Part model, mm, in its own coordinate system. A direction names the side the tool comes from. Coordinates: 2 decimals unless noted, no trailing zeros. Loops run counter-clockwise (first coordinate to the right, second up) from the corner with the lowest first, then second, coordinate; pieces in that order, holes last. Notation, with made-up numbers: M 9,47 L 62,47 A22 cw 62,59 Z; hole C 56.5,-28.75 d5. An arc over 180 degrees is marked long. Answer as a JSON object with one key per item and string values. Group by question number.
1. Saw through at B-B on z = 68.5. Write the cut outline in (x, y), then the cut area to 3 significant figures.
2. Saw through at C-C on z = 104. Write the cut outline in (x, y), then the cut area to 3 significant figures.
3. Drop flat-ended pins along their axis: pin 1 Ø5 at (x, z) = (-1, -143.5) entering from +Y; pin 2 Ø2 at (y, z) = (-1.5, 30.5) entering from +X; pin 3 Ø1.5 at (y, z) = (-4, -95.5) entering from -X. Give the stop position or say it passes through.
4. Saw through at A-A on x = 0. Write the cut outline in (y, z), then the cut area to 3 significant figures.
5. 3-axis set-ups, long thin cutter, end or side, ignore diameter. For faces 1 (the face through (11, 2, 74)), 2 (the face through (0, 8, -145)), 3 (the face through (11, 2, -74)), 4 (the face through (0, 0, 159)): which of +Z, -Z, +X, -X, +Y, -Y reach the whole face in a straight line?
6. Drill centre lines: L1, parallel to Z at x = 6, y = -13; L2, parallel to Y at x = 11.5, z = 42; L3, parallel to X at y = -4.75, z = -23.5. Where is each one in solid material? Low to high.
from build123d import *

# Parameters (mm, degrees)
BOSS_EXTRUDE1_DEPTH = 74
SKETCH2_R           = 10
BOSS_EXTRUDE2_DEPTH = 85
FILLET1_R           = 1
CUT_EXTRUDE1_DEPTH  = 2


with BuildPart() as part:
    # Sketch1 → Boss-Extrude1 (new, symmetric)
    with BuildSketch(Plane.XY):
        Polygon((16.500670693, 0), (8.250335347, 14.29), (-8.250335347, 14.29), (-16.500670693, 0), (-8.250335347, -14.29), (8.250335347, -14.29), align=None)
    extrude(amount=BOSS_EXTRUDE1_DEPTH, both=True)

    # Sketch2 → Boss-Extrude2 (add)
    with BuildSketch(Plane.XY.offset(74)):
        Circle(SKETCH2_R)
    boss_extrude2 = extrude(amount=BOSS_EXTRUDE2_DEPTH)

    # Mirror3: Boss-Extrude2 across plane
    add(boss_extrude2.mirror(Plane.XY))

    # Fillet1
    fillet1_edges = [part.edges().sort_by_distance(p)[0] for p in [
        (-10, 0, 74),
        (-10, 0, -74),
    ]]
    fillet(fillet1_edges, radius=FILLET1_R)

    # Sketch3 → Cut-Extrude1 (cut)
    with BuildSketch(Plane(origin=(0, 10, 0), x_dir=(1, 0, 0), z_dir=(0, 1, 0))):
        with BuildLine():
            Line((3, 133), (3, 159))
            Line((3, 159), (-3, 159))
            Line((-3, 159), (-3, 133))
            ThreePointArc((-3, 133), (0, 130), (3, 133))
        make_face()
    extrude(amount=-CUT_EXTRUDE1_DEPTH, mode=Mode.SUBTRACT)


solid = part.part
Outcome:
{
 "1": {"outline": "M -16.5,0 L -8.25,-14.29 L 8.25,-14.29 L 16.5,0 L 8.25,14.29 L -8.25,14.29 Z", "area": "707 mm²"},
 "2": {"outline": "C 0,0 d20", "area": "314 mm²"},
 "3": {"pin 1": "stops at y = 9.54", "pin 2": "stops at x = 16.21", "pin 3": "stops at x = -9.46"},
 "4": {"outline": "M -14.29,-74 L -11,-74 A1 cw -10,-75 L -10,-159 L 8,-159 L 8,-130 L 10,-130 L 10,-75 A1 cw 11,-74 L 14.29,-74 L 14.29,74 L 11,74 A1 cw 10,75 L 10,159 L -10,159 L -10,75 A1 cw -11,74 L -14.29,74 Z", "area": "7,570 mm²"},
 "5": {"face 1": "+Z", "face 2": "-Z, +Y", "face 3": "-Z", "face 4": "+Z, +X, -X, +Y, -Y"},
 "6": {"L1": "z = -74 to 74", "L2": "y = -8.66 to 8.66", "L3": "x = -13.76 to 13.76"}
}
